Could you check a few things on this model? Use its own coordinates, in mm. A direction names the side the tool comes from. Coordinates: 2 decimals unless noted, no trailing zeros. Loops run counter-clockwise (first coordinate to the right, second up) from the corner with the lowest first, then second, coordinate; pieces in that order, holes last. Notation, with made-up numbers: M -23,39.25 L 30,39.25 A25 ccw 30,73.25 Z; hole C 55.5,89.5 d7. An arc over 180 degrees is marked long. Write each question's results on one line, items separated by ' | '.
```python
from build123d import *

# Parameters (mm, degrees)
F0_R       = 21
F0_R_2     = 17.9
F1_DEPTH   = 5
F2_R       = 17.9
F3_DEPTH   = 5
F6_R       = 10
F7_DEPTH   = 25
F4_R       = 20
F7_FACE_R  = 10
F7_FACE1_R = 10


with BuildPart() as f1:
    # F0 (on Top) → F1 (new body)
    with BuildSketch(Plane.XY):
        Circle(F0_R)
        Circle(F0_R_2, mode=Mode.SUBTRACT)
        Circle(F0_R_2)
    extrude(amount=F1_DEPTH)

    # F2 (on face) → F3 (join)
    with BuildSketch(Plane.XY.offset(5)):
        Circle(F2_R)
    extrude(amount=F3_DEPTH)


with BuildPart() as f7:
    # F6 (on offset) → F7 (new body)
    with BuildSketch(Plane(origin=(0, 0, -25), x_dir=(1, 0, 0), z_dir=(0, 0, -1))):
        Circle(F6_R)
    extrude(amount=F7_DEPTH)

    # F10: sweep along a path in F9
    with BuildLine(Plane.XZ) as f10_path:
        Line((0, -50), (0, -58.9215382934))
        add(Plane.XZ * Edge.make_bspline(
            [(0, -58.9215382934), (0.244972108, -61.8164338234), (0.7711153536, -68.033997701), (-4.6363235106, -79.4328354028), (-19.6589254166, -90.9882543348), (-29.0378853679, -98.2025712729)],
            knots=[0, 0, 0, 0, 0.2465968941, 0.529632909, 1, 1, 1, 1], degree=3))
    # F7_face1 (on face) → F10 (sweep)
    with BuildSketch(Plane(origin=(0, 0, -50), x_dir=(1, 0, 0), z_dir=(0, 0, -1))):
        Circle(F7_FACE1_R)
    sweep(path=f10_path.line, transition=Transition.RIGHT)


with BuildPart() as f8:
    # F4 (on face) → F8 section 0
    with BuildSketch(Plane(origin=(0, 0, 0), x_dir=(1, 0, 0), z_dir=(0, 0, -1))):
        Circle(F4_R)
    # F7_face (on face) → F8 section 1
    with BuildSketch(Plane.XY.offset(-25)):
        Circle(F7_FACE_R)
    loft()


solid = f1.part
```
(1) Imagine slicing it at D-D, the plane z = 7.5. List the corners of the cut face in (x, y) for me, and give its area (3 significant figures).
Reported:
outline: C 0,0 d35.8 | area: 1,010 mm2
(2) Will these pins go through, and if not, where does the flat tip stop? P1, Ø4, axis at x = 4, z = 4.5, coming from the +Y side; P2, Ø1.5, axis at y = 5.5, z = 8.5, coming from the +X side.
Reported:
P1: stops at y = 20.9 | P2: stops at x = 17.26
(3) Please list where these lines run through material, in increasing order: probe 1 along Y at (x, z) = (-11, 3.75); probe 2 along Z at (x, y) = (-13, 15); probe 3 along X at (y, z) = (11, 8.25). Write a range as from..to.
Reported:
probe 1: y = -17.89..17.89 | probe 2: z = 0..5 | probe 3: x = -14.12..14.12
(4) Imagine slicing it at A-A, the plane x = 0. List the corners of the cut face in (y, z) for me, and give its area (3 significant figures).
Reported:
outline: M -21,0 L 21,0 L 21,5 L 17.9,5 L 17.9,10 L -17.9,10 L -17.9,5 L -21,5 Z | area: 389 mm2
(5) Which directions (+Z, -Z, +X, -X, +Y, -Y) give clear straight access to the entire face, cutting with the end or side of a thin tool? Please do faces 1 (the flat face through (0, 0, 0)), 2 (the flat face through (15.5, 9.4, 5)).
Reported:
face 1: -Z, +X, -X, +Y, -Y | face 2: +Z
(6) Imagine slicing it at C-C, the plane z = 1.5. List the corners of the cut face in (x, y) for me, and give its area (3 significant figures).
Reported:
outline: C 0,0 d42 | area: 1,390 mm2
